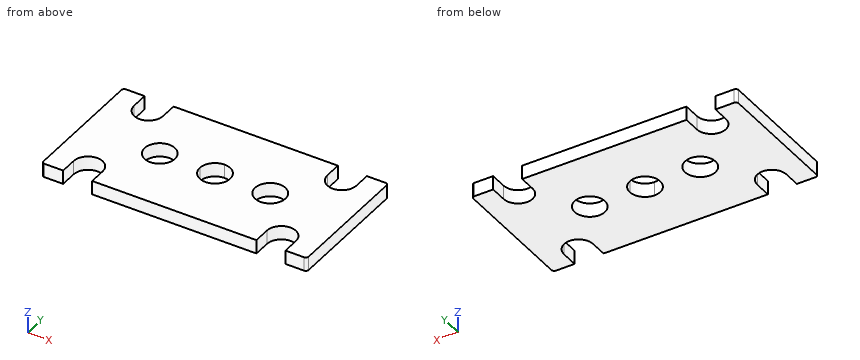
from build123d import *

# Parameters (mm, degrees)
SKETCH_1_W          = 96
SKETCH_1_H          = 47
EXTRUDE_1_DEPTH     = 5
FILLET_1_R          = 1
CUT_EXTRUDE_2_DEPTH = 10
SKETCH_2_R          = 5.25
CUT_EXTRUDE_3_DEPTH = 10


with BuildPart() as part:
    # 草图1 → 凸台-拉伸1 (new body)
    with BuildSketch(Plane.XY):
        with Locations((48, -23.5)):
            Rectangle(SKETCH_1_W, SKETCH_1_H)
    extrude(amount=EXTRUDE_1_DEPTH)

    # 圆角1
    fillet_1_edges = [part.edges().sort_by_distance(p)[0] for p in [
        (0, 0, 2.5),
        (96, 0, 2.5),
        (96, -47, 2.5),
        (0, -47, 2.5),
    ]]
    fillet(fillet_1_edges, radius=FILLET_1_R)

    # 草图8 → 切除-拉伸2 (cut)
    with BuildSketch(Plane.XY.offset(5)):
        with BuildLine():
            ThreePointArc((22.5, -23.5), (28, -29), (33.5, -23.5))
            Line((33.5, -23.5), (22.5, -23.5))
        make_face()
        with BuildLine():
            Line((22.5, -23.5), (33.5, -23.5))
            ThreePointArc((33.5, -23.5), (28, -18), (22.5, -23.5))
        make_face()
        with BuildLine():
            ThreePointArc((42.5, -23.5), (44.110912703, -27.389087297), (48, -29))
            Line((48, -29), (48, -23.5))
            Line((48, -23.5), (42.5, -23.5))
        make_face()
        with BuildLine():
            Line((48, -23.5), (48, -29))
            ThreePointArc((48, -29), (51.889087297, -27.389087297), (53.5, -23.5))
            Line((53.5, -23.5), (48, -23.5))
        make_face()
        with BuildLine():
            Line((42.5, -23.5), (48, -23.5))
            Line((48, -23.5), (48, -18))
            ThreePointArc((48, -18), (44.110912703, -19.610912703), (42.5, -23.5))
        make_face()
        with BuildLine():
            Line((48, -18), (48, -23.5))
            Line((48, -23.5), (53.5, -23.5))
            ThreePointArc((53.5, -23.5), (51.889087297, -19.610912703), (48, -18))
        make_face()
        with BuildLine():
            ThreePointArc((73.5, -23.5), (68, -18), (62.5, -23.5))
            Line((62.5, -23.5), (73.5, -23.5))
        make_face()
        with BuildLine():
            Line((73.5, -23.5), (62.5, -23.5))
            ThreePointArc((62.5, -23.5), (68, -29), (73.5, -23.5))
        make_face()
    extrude(amount=-CUT_EXTRUDE_2_DEPTH, mode=Mode.SUBTRACT)

    # 草图2 → 切除-拉伸3 (cut)
    with BuildSketch(Plane.XY.offset(5)):
        with Locations((83, -6)):
            Circle(SKETCH_2_R)
        with Locations((13, -6)):
            Circle(SKETCH_2_R)
        with Locations((13, -41)):
            Circle(SKETCH_2_R)
        with Locations((83, -41)):
            Circle(SKETCH_2_R)
        with BuildLine():
            Line((18.25, -6), (18.25, 0))
            Line((18.25, 0), (7.75, 0))
            Line((7.75, 0), (7.75, -6))
            ThreePointArc((7.75, -6), (13, -0.75), (18.25, -6))
        make_face()
        with BuildLine():
            Line((7.75, -47), (18.25, -47))
            Line((18.25, -47), (18.25, -41))
            ThreePointArc((18.25, -41), (13, -46.25), (7.75, -41))
            Line((7.75, -41), (7.75, -47))
        make_face()
        with BuildLine():
            Line((77.75, -41), (77.75, -47))
            Line((77.75, -47), (88.25, -47))
            Line((88.25, -47), (88.25, -41))
            ThreePointArc((88.25, -41), (83, -46.25), (77.75, -41))
        make_face()
        with BuildLine():
            Line((88.25, 0), (77.75, 0))
            Line((77.75, 0), (77.75, -6))
            ThreePointArc((77.75, -6), (83, -0.75), (88.25, -6))
            Line((88.25, -6), (88.25, 0))
        make_face()
    extrude(amount=-CUT_EXTRUDE_3_DEPTH, mode=Mode.SUBTRACT)


solid = part.part
Model file for the job. Use its own axes, mm. Coordinates: 2 decimals unless noted, no trailing zeros. Loops run counter-clockwise (first coordinate to the right, second up) from the corner with the lowest first, then second, coordinate; pieces in that order, holes last. Notation, with made-up numbers: (-35, -35.75) -> (-30, -35.75) arc R11 cw to (-30, -14.75) -> close; hole circle Ø9 at (35.5, 40.5). An arc over 180 degrees is marked (long way). Use one line per item in the form item = value. Start each with the question number.
(1) Cut at D-D on y = -27.5. Give the cut face in (x, z), and give its area (3 significant figures).
(2) Cut at C-C on z = 3.7. Give the cut face in (x, y), and give its area (3 significant figures).
(3) Cut at A-A on y = -44. Give the cut face in (x, z).
(4) Cut at B-B on x = 68. Give the cut face in (y, z), and give its area (3 significant figures).
(5) Probe probe 1 along X at (y, z) = (-41.5, 0.8); probe 2 along X at (y, z) = (-28, 3.55); probe 3 along Y at (x, z) = (68, 1.85). List the from-to ranges inside material, lowest first. Write a range as from..to.
Values:
q1.outline = (0, 0) -> (24.23, 0) -> (24.23, 5) -> (0, 5) -> close; (31.77, 0) -> (44.23, 0) -> (44.23, 5) -> (31.77, 5) -> close; (51.77, 0) -> (64.23, 0) -> (64.23, 5) -> (51.77, 5) -> close; (71.77, 0) -> (96, 0) -> (96, 5) -> (71.77, 5) -> close
q1.area = 367 mm2
q2.outline = (0, -46) arc R1 ccw to (1, -47) -> (7.75, -47) -> (7.75, -41) arc R5.25 cw to (18.25, -41) -> (18.25, -47) -> (77.75, -47) -> (77.75, -41) arc R5.25 cw to (88.25, -41) -> (88.25, -47) -> (95, -47) arc R1 ccw to (96, -46) -> (96, -1) arc R1 ccw to (95, 0) -> (88.25, 0) -> (88.25, -6) arc R5.25 cw to (77.75, -6) -> (77.75, 0) -> (18.25, 0) -> (18.25, -6) arc R5.25 cw to (7.75, -6) -> (7.75, 0) -> (1, 0) arc R1 ccw to (0, -1) -> close; hole circle Ø11 at (28, -23.5); hole circle Ø11 at (48, -23.5); hole circle Ø11 at (68, -23.5)
q2.area = 3,800 mm2
q3.outline = (0, 0) -> (7.75, 0) -> (7.75, 5) -> (0, 5) -> close; (18.25, 0) -> (77.75, 0) -> (77.75, 5) -> (18.25, 5) -> close; (88.25, 0) -> (96, 0) -> (96, 5) -> (88.25, 5) -> close
q4.outline = (-47, 0) -> (-29, 0) -> (-29, 5) -> (-47, 5) -> close; (-18, 0) -> (0, 0) -> (0, 5) -> (-18, 5) -> close
q4.area = 180 mm2
q5.probe_1 = 0..7.75, 18.25..77.75, 88.25..96
q5.probe_2 = 0..24.84, 31.16..44.84, 51.16..64.84, 71.16..96
q5.probe_3 = -47..-29, -18..0
